from build123d import *

# Parameters (mm, degrees)
F0_R     = 13.2
F0_R_2   = 11.2
F1_DEPTH = 7
F1_TAPER = -3


with BuildPart() as f1:
    # F0 (on Top) → F1 (new body)
    with BuildSketch(Plane.XY):
        with BuildLine():
            ThreePointArc((10.9010818376, 19.4378948031), (0.0215551002, 13.6814609359), (-10.8767136673, 19.4023324402))
            ThreePointArc((-10.8767136673, 19.4023324402), (-11.7146747863, 6.3266103812), (-23.0513772317, -0.2427019014))
            ThreePointArc((-23.0513772317, -0.2427019014), (-13.8657154546, -4.1881001415), (-10.0800128199, -13.4407216683))
            ThreePointArc((-10.0800128199, -13.4407216683), (-10.4709476124, -16.6294280689), (-11.6205959274, -19.6292592764))
            ThreePointArc((-11.6205959274, -19.6292592764), (-0.9162642999, -13.4149873045), (10.7426883573, -17.5705516067))
            ThreePointArc((10.7426883573, -17.5705516067), (12.4749250479, -5.858500474), (22.8996505618, -0.2462029369))
            ThreePointArc((22.8996505618, -0.2462029369), (11.7615752414, 6.4634627634), (10.9010818376, 19.4378948031))
        make_face()
        Circle(F0_R, mode=Mode.SUBTRACT)
        with BuildLine():
            ThreePointArc((36.4800128199, -13.4407216683), (32.4783609921, -3.9733888389), (22.8996505618, -0.2462029369))
            ThreePointArc((22.8996505618, -0.2462029369), (12.4749250479, -5.858500474), (10.7426883573, -17.5705516067))
            ThreePointArc((10.7426883573, -17.5705516067), (12.8230245623, -20.1337465562), (14.2794462685, -23.096279744))
            ThreePointArc((14.2794462685, -23.096279744), (28.5446363355, -25.5454207244), (36.4800128199, -13.4407216683))
        make_face()
        with Locations((23.2800128199, -13.4407216683)):
            Circle(F0_R_2, mode=Mode.SUBTRACT)
        with BuildLine():
            ThreePointArc((10.9010818376, 19.4378948031), (12.6121822112, 22.9862078018), (13.2, 26.8814433366))
            ThreePointArc((13.2, 26.8814433366), (-3.9158255574, 39.48724796), (-10.8767136673, 19.4023324402))
            ThreePointArc((-10.8767136673, 19.4023324402), (0.0215551002, 13.6814609359), (10.9010818376, 19.4378948031))
        make_face()
        with Locations((0, 26.8814433366)):
            Circle(F0_R_2, mode=Mode.SUBTRACT)
        with BuildLine():
            ThreePointArc((-10.0800128199, -13.4407216683), (-13.8657154546, -4.1881001415), (-23.0513772317, -0.2427019014))
            ThreePointArc((-23.0513772317, -0.2427019014), (-35.0600457348, -19.3964604574), (-12.5159396425, -21.0810573043))
            ThreePointArc((-12.5159396425, -21.0810573043), (-12.0893262179, -20.3421712665), (-11.6205959274, -19.6292592764))
            ThreePointArc((-11.6205959274, -19.6292592764), (-10.4709476124, -16.6294280689), (-10.0800128199, -13.4407216683))
        make_face()
        with Locations((-23.2800128199, -13.4407216683)):
            Circle(F0_R_2, mode=Mode.SUBTRACT)
    extrude(amount=F1_DEPTH, taper=F1_TAPER)


solid = f1.part
Part model, mm, in its own coordinate system. Coordinates: 2 decimals unless noted, no trailing zeros. Put each result on its own line as item: value.
1. Flat gauge pins, fed straight in: pin 1 Ø1.5 at (y, z) = (-19.5, 3.5) entering from -X; pin 2 Ø3 at (x, z) = (7.5, 3) entering from -Y. Where does each tip first touch, or does it go through?
Final values:
pin 1: stops at x = -35.57
pin 2: stops at y = -16.3
2. Band-saw the part on A-A (z = 2.25). Give the number of separate pieces and of enclosed holes in the cut face, then the cut area to 3 significant figures.
Final values:
separate pieces: 1
enclosed holes: 4
area: 720 mm²
3. Two-plate mould, pull along X, no slides. Class faces 1 (the conical face through (-12.8, -16.7, 4.3)), 2 (the conical face through (-2.379, 37.594, 4.327)), 3 (the flat face through (12, 5, 7)): +X half, -X half, draft (parallel to the pull), parting line (faces both ways), or undercut.
Final values:
face 1: undercut
face 2: undercut
face 3: draft
4. Probe line 1 along X through (y, z) = (-6, 2.5); line 2 along X through (y, z) = (-22.5, 0.5); line 3 along Y through (x, z) = (7.5, 1.25). List the from-to ranges inside material, lowest first. Write a range as [from, to].
Final values:
line 1: x = [-34.34, -31.48], [-15.09, -11.61], [11.61, 15.09], [31.48, 34.34]
line 2: x = [-32.92, -29.82], [-16.74, -13.64], [14.02, 16.74], [29.82, 32.92]
line 3: y = [-15.24, -10.78], [10.78, 18.65], [35.11, 37.82]
